The listing builds one solid part. Answer for the finished solid, in the listing's coordinates (mm). A direction names the side the tool comes from. Give positions to 0.01 mm unless a question says otherwise; leave off trailing zeros. Write each loop counter-clockwise with the first axis right and the second up, starting at its lowest first coordinate (ties: lowest second). Pieces come first, ordered by that corner, then holes. Notation, with made-up numbers: (-7.75, 33.25) - (40.25, 33.25) arc R21 cw to (40.25, 54.25) - close; hole circle Ø8 at (4, -29.75). An arc over 180 degrees is marked (long way). Answer as CSV lines item,"result". Start each with the question number.
(1) For a pull along X with two mould halves and no side action, classify faces 1 (the face through (4.75, 0.03, 2.24)), 2 (the face through (-8.89, 1.31, -1.11)), 3 (the face through (0, 0, -1.905)) as pulls with the +X half, pulls with the -X half, needs draft (parallel to the pull), parting line crosses it, or undercut.
(2) Find section C-C (z = 23). Write down the section's boundary in (x, y), then the cut area to 3 significant figures.
(3) Straight lines are drawn through the part: probe 1 along Y at (x, z) = (0, 0.4); probe 2 along Y at (x, z) = (0, 0.55); probe 3 along Z at (x, y) = (0.5, 9.75). For each, find the intervals that lie inside material, in ascending order.
(4) Each of these flat-tipped pins is pushed along its axis until it touches: pin 1 Ø3 at (x, y) = (0, 0) entering from +Z; pin 2 Ø3 at (x, z) = (4, 43) entering from -Y; pin 3 Ø0.8 at (y, z) = (0, 0.5) entering from -X. Where does it stop, or does it pass through?
(5) For faces 4 (the face through (-8.836, 1.816, -1.114)), 5 (the face through (-8.83, -3.524, 0.261)), 6 (the face through (0, 0, 51.5)), determine the directions among +Z, -Z, +X, -X, +Y, -Y from which every point of the face is accessible in a straight line to the end or side of a thin tool.
(6) Find section A-A (z = 49). Write down the section's boundary in (x, y) (3 decimals).
(7) Find section B-B (z = 41). Write down the section's boundary in (x, y) (3 decimals).
from build123d import *

# Parameters (mm, degrees)
SKETCH1_R                 = 12.05
BOSS_EXTRUDE1_DEPTH       = 30.75
FILLET2_R                 = 1
SKETCH2_R                 = 12.375
BOSS_EXTRUDE2_DEPTH       = 20.75
SKETCH3_R                 = 3.5
SKETCH3_R_2               = 2
BOSS_EXTRUDE3_DEPTH       = 2.375
CHAMFER1_SIZE             = 0.254
M3X0_5_TAPPED_HOLE1_D     = 2.5
M3X0_5_TAPPED_HOLE1_DEPTH = 7.5
M3X0_5_TAPPED_HOLE1_TIP   = 0.751075774
SKETCH7_R                 = 11.8
CUT_EXTRUDE1_DEPTH        = 0.762
SKETCH8_R                 = 4.5
BOSS_EXTRUDE4_DEPTH       = 0.254
BOSS_EXTRUDE4_TAPER       = 60
SKETCH9_R                 = 3.1875
BOSS_EXTRUDE5_DEPTH       = 2.413
FILLET1_R                 = 0.254
SKETCH10_R                = 1.524
BOSS_EXTRUDE6_DEPTH       = 1.016
BOSS_EXTRUDE7_DEPTH       = 3.175
SKETCH12_R                = 0.635
CUT_EXTRUDE2_DEPTH        = 3.175
CHAMFER2_SIZE             = 0.635
BOSS_EXTRUDE8_DEPTH       = 1.016
CUT_EXTRUDE3_DEPTH        = 10
CUT_EXTRUDE3_DEPTH_BACK   = 3
SKETCH15_R                = 1
BOSS_EXTRUDE9_DEPTH       = 0.5


with BuildPart() as part:
    # Sketch1 → Boss-Extrude1 (new body)
    with BuildSketch(Plane.XY):
        Circle(SKETCH1_R)
    extrude(amount=BOSS_EXTRUDE1_DEPTH)

    # Fillet2
    fillet2_edges = [part.edges().sort_by_distance(p)[0] for p in [
        (-12.05, 0, 30.75),
    ]]
    fillet(fillet2_edges, radius=FILLET2_R)

    # Sketch2 → Boss-Extrude2 (add)
    with BuildSketch(Plane.XY.offset(30.75)):
        Circle(SKETCH2_R)
    extrude(amount=BOSS_EXTRUDE2_DEPTH)

    # Sketch3 → Boss-Extrude3 (add)
    with BuildSketch(Plane.XY.offset(51.5)):
        Circle(SKETCH3_R)
        Circle(SKETCH3_R_2, mode=Mode.SUBTRACT)
    extrude(amount=BOSS_EXTRUDE3_DEPTH)

    # Chamfer1
    chamfer1_edges = [part.edges().sort_by_distance(p)[0] for p in [
        (-3.5, 0, 53.875),
        (-2, 0, 53.875),
    ]]
    chamfer(chamfer1_edges, length=CHAMFER1_SIZE)

    # M3x0.5 Tapped Hole1
    with Locations(Plane.XY.offset(51.5)):
        with Locations((-8.5, 0), (8.5, 0)):
            Hole(M3X0_5_TAPPED_HOLE1_D / 2, depth=M3X0_5_TAPPED_HOLE1_DEPTH)
            with Locations((0, 0, -(M3X0_5_TAPPED_HOLE1_DEPTH + M3X0_5_TAPPED_HOLE1_TIP / 2))):  # 118° drill point
                Cone(0, M3X0_5_TAPPED_HOLE1_D / 2, M3X0_5_TAPPED_HOLE1_TIP, mode=Mode.SUBTRACT)

    # Sketch7 → Cut-Extrude1 (cut)
    with BuildSketch(Plane(origin=(0, 0, 0), x_dir=(-1, 0, 0), z_dir=(0, 0, -1))):
        Circle(SKETCH7_R)
    extrude(amount=-CUT_EXTRUDE1_DEPTH, mode=Mode.SUBTRACT)

    # Sketch8 → Boss-Extrude4 (add)
    with BuildSketch(Plane(origin=(0, 0, 0.762), x_dir=(-1, 0, 0), z_dir=(0, 0, -1))):
        Circle(SKETCH8_R)
    extrude(amount=BOSS_EXTRUDE4_DEPTH, taper=BOSS_EXTRUDE4_TAPER)

    # Sketch9 → Boss-Extrude5 (add)
    with BuildSketch(Plane(origin=(0, 0, 0.508), x_dir=(-1, 0, 0), z_dir=(0, 0, -1))):
        Circle(SKETCH9_R)
    extrude(amount=BOSS_EXTRUDE5_DEPTH)

    # Fillet1
    fillet1_edges = [part.edges().sort_by_distance(p)[0] for p in [
        (3.1875, 0, 0.508),
        (3.1875, 0, -1.905),
    ]]
    fillet(fillet1_edges, radius=FILLET1_R)

    # Sketch10 → Boss-Extrude6 (add)
    with BuildSketch(Plane(origin=(0, 0, 0.762), x_dir=(-1, 0, 0), z_dir=(0, 0, -1))):
        with Locations((8.863269777, 1.562833599)):
            Circle(SKETCH10_R)
        with Locations((-8.863269777, -1.562833599)):
            Circle(SKETCH10_R)
    extrude(amount=BOSS_EXTRUDE6_DEPTH)

    # Sketch11 → Boss-Extrude7 (add)
    with BuildSketch(Plane(origin=(0, 0, -0.254), x_dir=(-1, 0, 0), z_dir=(0, 0, -1))):
        Polygon((-10.007333694, -2.022481295), (-7.630992586, -1.603468242), (-7.71920586, -1.103185903), (-10.095546968, -1.522198956), align=None)
        Polygon((7.71920586, 1.103185903), (10.095546968, 1.522198956), (10.007333694, 2.022481295), (7.630992586, 1.603468242), align=None)
    extrude(amount=BOSS_EXTRUDE7_DEPTH)

    # Sketch12 → Cut-Extrude2 (cut)
    with BuildSketch(Plane(origin=(0.044106637, 0.250141169, 0), x_dir=(0.984807753, -0.173648178, 0), z_dir=(0.173648178, 0.984807753, 0))):
        with Locations((-9, 2.159)):
            Circle(SKETCH12_R)
        with Locations((9, 2.159)):
            Circle(SKETCH12_R)
    extrude(amount=-CUT_EXTRUDE2_DEPTH, mode=Mode.SUBTRACT)

    # Chamfer2
    chamfer2_edges = [part.edges().sort_by_distance(p)[0] for p in [
        (-7.675099223, 1.353327073, -3.429),
        (-10.051440331, 1.772340125, -3.429),
        (10.051440331, -1.772340125, -3.429),
        (7.675099223, -1.353327073, -3.429),
    ]]
    chamfer(chamfer2_edges, length=CHAMFER2_SIZE)

    # Sketch13 → Boss-Extrude8 (add)
    with BuildSketch(Plane(origin=(0, 0, 0.762), x_dir=(-1, 0, 0), z_dir=(0, 0, -1))):
        with BuildLine():
            Line((-7.339269777, 2), (-7.339269777, -2))
            ThreePointArc((-7.339269777, -2), (-8.863269777, -3.524), (-10.387269777, -2))
            Line((-10.387269777, -2), (-10.387269777, 2))
            ThreePointArc((-10.387269777, 2), (-8.863269777, 3.524), (-7.339269777, 2))
        make_face()
        with BuildLine():
            Line((7.339269777, 2), (7.339269777, -2))
            ThreePointArc((7.339269777, -2), (8.863269777, -3.524), (10.387269777, -2))
            Line((10.387269777, -2), (10.387269777, 2))
            ThreePointArc((10.387269777, 2), (8.863269777, 3.524), (7.339269777, 2))
        make_face()
    extrude(amount=BOSS_EXTRUDE8_DEPTH)

    # Sketch14 → Cut-Extrude3 (cut, two sides)
    with BuildSketch(Plane(origin=(0, 0, 0.762), x_dir=(-1, 0, 0), z_dir=(0, 0, -1))) as cut_extrude3_sk:
        with BuildLine():
            ThreePointArc((-4.113620668, 2.375), (-4.75, 0), (-4.113620668, -2.375))
            ThreePointArc((-4.113620668, -2.375), (-3.772114317, -2.466506351), (-3.680607966, -2.125))
            ThreePointArc((-3.680607966, -2.125), (-4.25, 0), (-3.680607966, 2.125))
            ThreePointArc((-3.680607966, 2.125), (-3.772114317, 2.466506351), (-4.113620668, 2.375))
        make_face()
        with BuildLine():
            ThreePointArc((4.113620668, -2.375), (4.75, 0), (4.113620668, 2.375))
            ThreePointArc((4.113620668, 2.375), (3.772114317, 2.466506351), (3.680607966, 2.125))
            ThreePointArc((3.680607966, 2.125), (4.25, 0), (3.680607966, -2.125))
            ThreePointArc((3.680607966, -2.125), (3.772114317, -2.466506351), (4.113620668, -2.375))
        make_face()
    extrude(amount=CUT_EXTRUDE3_DEPTH, mode=Mode.SUBTRACT)
    extrude(cut_extrude3_sk.sketch, amount=-CUT_EXTRUDE3_DEPTH_BACK, mode=Mode.SUBTRACT)

    # Sketch15 → Boss-Extrude9 (add)
    with BuildSketch(Plane(origin=(0, 0, 0.762), x_dir=(-1, 0, 0), z_dir=(0, 0, -1))):
        with Locations((-8.191520443, 5.735764364)):
            Circle(SKETCH15_R)
        with Locations((8.191520443, 5.735764364)):
            Circle(SKETCH15_R)
        with Locations((8.191520443, -5.735764364)):
            Circle(SKETCH15_R)
        with Locations((-8.191520443, -5.735764364)):
            Circle(SKETCH15_R)
    extrude(amount=BOSS_EXTRUDE9_DEPTH)


solid = part.part
Result set:
1,face 1,"undercut"
1,face 2,"pulls with the -X half"
1,face 3,"needs draft"
2,outline,"circle Ø24.1 at (0, 0)"
2,area,"456 mm^2"
3,probe 1,"-12.05 to -11.8, -3.23 to 3.23, 11.8 to 12.05"
3,probe 2,"-12.05 to -11.8, -4.13 to 4.13, 11.8 to 12.05"
3,probe 3,"0.76 to 51.5"
4,pin 1,"z = 51.5"
4,pin 2,"y = -12.12"
4,pin 3,"x = -12.05"
5,face 4,"-Z, +Y"
5,face 5,"-Z"
5,face 6,"+Z"
6,outline,"circle Ø24.75 at (0, 0); hole circle Ø2.5 at (-8.5, 0); hole circle Ø2.5 at (8.5, 0)"
7,outline,"circle Ø24.75 at (0, 0)"
